```python
from build123d import *

# Parameters (mm, degrees)
SKETCH1_W           = 87
SKETCH1_H           = 127
SKETCH1_W_2         = 79
SKETCH1_H_2         = 119
SKETCH1_W_3         = 63
SKETCH1_H_3         = 107
BOSS_EXTRUDE1_DEPTH = 3
CHAMFER2_SIZE       = 3
FILLET1_R           = 1


with BuildPart() as part:
    # Sketch1 → Boss-Extrude1 (new body)
    # profile 1 of 2: a face of its own
    with BuildSketch(Plane.XY):
        with Locations((191.590301411, -234.498578163)):
            Rectangle(SKETCH1_W, SKETCH1_H)
        with Locations((191.590301411, -234.498578163)):
            Rectangle(SKETCH1_W_2, SKETCH1_H_2, mode=Mode.SUBTRACT)
    # profile 2 of 2: a face of its own
    with BuildSketch(Plane.XY):
        with Locations((191.590301411, -234.498578163)):
            Rectangle(SKETCH1_W_2, SKETCH1_H_2)
        with Locations((190.590301411, -232.498578163)):
            Rectangle(SKETCH1_W_3, SKETCH1_H_3, mode=Mode.SUBTRACT)
    extrude(amount=BOSS_EXTRUDE1_DEPTH)

    # Chamfer2
    chamfer2_edges = [part.edges().sort_by_distance(p)[0] for p in [
        (190.590301411, -285.998578163, 3),
        (159.090301411, -232.498578163, 3),
        (190.590301411, -178.998578163, 3),
        (222.090301411, -232.498578163, 3),
    ]]
    chamfer(chamfer2_edges, length=CHAMFER2_SIZE - 0.0001)  # a hair under: the kernel refuses the full size

    # Fillet1
    fillet1_edges = [part.edges().sort_by_distance(p)[0] for p in [
        (191.590301411, -170.998578163, 3),
        (148.090301411, -234.498578163, 3),
        (191.590301411, -297.998578163, 3),
        (235.090301411, -234.498578163, 3),
    ]]
    fillet(fillet1_edges, radius=FILLET1_R)


solid = part.part
```
Read the model definition and answer for the solid it produces. Units are mm, in the model's axes. A direction names the side the tool comes from. Round coordinates to 2 decimals unless told otherwise and drop trailing zeros. Write each loop counter-clockwise with the first axis right and the second up, starting at its lowest first coordinate (ties: lowest second). Pieces come first, ordered by that corner, then holes. Notation, with made-up numbers: (-16.5, 22) -> (9.5, 22) arc R18 ccw to (9.5, 42) -> close; hole circle Ø7 at (77, 42.5). An arc over 180 degrees is marked (long way). Answer in a Markdown table with one row per item. Add a question column.
1) Determine the mould class of faces 1 (the face through (223.61, -233.29, 1.52)), 2 (the face through (190, -288, 2)), 3 (the face through (226, -230, 3)) for opening direction X: pulls with the +X half, pulls with the -X half, needs draft (parallel to the pull), parting line crosses it, or undercut.
2) Which of the six approach directions +Z, -Z, +X, -X, +Y, -Y give full straight-line access (tool end or side, diameter ignored) to faces 4 (the face through (152, -234, 0)), 5 (the face through (157.57, -233.29, 1.52))?
3) Given P1, Ø3, axis at x = 172, y = -284, coming from the -Z side, flat-ended and moving along its own axis, determine where the tip first touches the part or whether it passes through.
4) Find section C-C, the plane z = 0.6. Determine the outline of the cut face in (x, y).
5) Consider line 1 (X direction, y = -188, z = 0.2); line 2 (Y direction, x = 219.5, z = 2.7); line 3 (X direction, y = -237, z = 1.1). Determine where each line is inside the solid, lowest interval first.
Findings below:
| question | item | result |
|---|---|---|
| 1 | face 1 | undercut |
| 1 | face 2 | undercut |
| 1 | face 3 | needs draft |
| 2 | face 4 | -Z, +X, -X, +Y, -Y |
| 2 | face 5 | +Z |
| 3 | P1 | through |
| 4 | outline | (148.09, -298) -> (235.09, -298) -> (235.09, -171) -> (148.09, -171) -> close; hole (158.49, -286.6) -> (222.69, -286.6) -> (222.69, -178.4) -> (158.49, -178.4) -> close |
| 5 | line 1 | 148.09 to 158.89, 222.29 to 235.09 |
| 5 | line 2 | -297.71 to -288.7, -176.3 to -171.28 |
| 5 | line 3 | 148.09 to 157.99, 223.19 to 235.09 |
